from build123d import *

# Parameters (mm, degrees)
F0_R     = 3.175
F1_DEPTH = 3.048


with BuildPart() as f1:
    # F0 (on Front) → F1 (new body)
    with BuildSketch(Plane.XZ):
        with BuildLine():
            ThreePointArc((-9.4236638917, 68.6386150491), (-0.6947036893, 57.753275869), (9.525, 67.252908061))
            ThreePointArc((9.525, 67.252908061), (9.5066279666, 67.8442199118), (9.4515827392, 68.4332506914))
            ThreePointArc((9.4515827392, 68.4332506914), (0.1036267117, 76.7773443438), (-9.4236638917, 68.6386150491))
        make_face()
        with Locations((0, 67.252908061)):
            Circle(F0_R, mode=Mode.SUBTRACT)
        with BuildLine():
            ThreePointArc((9.4515827392, 68.4332506914), (9.5066279666, 67.8442199118), (9.525, 67.252908061))
            ThreePointArc((9.525, 67.252908061), (-0.6947036893, 57.753275869), (-9.4236638917, 68.6386150491))
            Line((-9.4236638917, 68.6386150491), (-17.0751139076, 16.6040263124))
            Line((-17.0751139076, 16.6040263124), (-9.4598263283, -48.1594366871))
            ThreePointArc((-9.4598263283, -48.1594366871), (-0.5571262079, -37.5383993165), (9.525, -47.047091939))
            ThreePointArc((9.525, -47.047091939), (6.9705567315, -53.5383910272), (0.6773435479, -56.5479777249))
            Line((0.6773435479, -56.5479777249), (44.7324052746, -54.9795665535))
            ThreePointArc((44.7324052746, -54.9795665535), (36.5125000006, -47.0471928378), (44.7322036046, -39.1146101473))
            Line((44.7322036046, -39.1146101473), (18.9234018404, -38.1964439189))
            ThreePointArc((18.9234018404, -38.1964439189), (13.2224661173, -35.485992741), (11.2938088242, -29.4753775685))
            Line((11.2938088242, -29.4753775685), (15.4327477068, 12.7318970133))
            ThreePointArc((15.4327477068, 12.7318970133), (-15.8733066778, 16.6847703328), (15.5348463028, 19.7215737442))
            Line((15.5348463028, 19.7215737442), (9.4515827392, 68.4332506914))
        make_face()
        with Locations((-3.175, 52.978108061)):
            Circle(F0_R, mode=Mode.SUBTRACT)
        with BuildLine():
            Line((15.8615962708, 17.1051263858), (15.5348463028, 19.7215737442))
            ThreePointArc((15.5348463028, 19.7215737442), (-15.8733066778, 16.6847703328), (15.4327477068, 12.7318970133))
            Line((15.4327477068, 12.7318970133), (15.8615962708, 17.1051263858))
        make_face()
        with Locations((0, 16.452908061)):
            Circle(F0_R, mode=Mode.SUBTRACT)
        with BuildLine():
            ThreePointArc((15.8615962708, 17.1051263858), (15.7526378986, 18.4201457783), (15.5348463028, 19.7215737442))
            Line((15.5348463028, 19.7215737442), (15.8615962708, 17.1051263858))
        make_face()
        with BuildLine():
            ThreePointArc((15.875, 16.452908061), (15.871648714, 16.7790860811), (15.8615962708, 17.1051263858))
            Line((15.8615962708, 17.1051263858), (15.4327477068, 12.7318970133))
            ThreePointArc((15.4327477068, 12.7318970133), (15.7640492077, 14.5793078964), (15.875, 16.452908061))
        make_face()
        with BuildLine():
            ThreePointArc((9.525, -47.047091939), (-0.5571262079, -37.5383993165), (-9.4598263283, -48.1594366871))
            ThreePointArc((-9.4598263283, -48.1594366871), (-6.329713314, -54.1647006921), (0, -56.572091939))
            Line((0, -56.572091939), (0.6773435479, -56.5479777249))
            ThreePointArc((0.6773435479, -56.5479777249), (6.9705567315, -53.5383910272), (9.525, -47.047091939))
        make_face()
        with Locations((0, -47.047091939)):
            Circle(F0_R, mode=Mode.SUBTRACT)
        with BuildLine():
            Line((0.6773435479, -56.5479777249), (0, -56.572091939))
            ThreePointArc((0, -56.572091939), (0.3388863295, -56.5660614764), (0.6773435479, -56.5479777249))
        make_face()
        with BuildLine():
            ThreePointArc((52.3875, -47.047091939), (50.1615627179, -41.5351088503), (44.7322036046, -39.1146101473))
            ThreePointArc((44.7322036046, -39.1146101473), (36.5125000006, -47.0471928378), (44.7324052746, -54.9795665535))
            ThreePointArc((44.7324052746, -54.9795665535), (50.1616327839, -52.5590024237), (52.3875, -47.047091939))
        make_face()
        with Locations((44.45, -47.047091939)):
            Circle(F0_R, mode=Mode.SUBTRACT)
    extrude(amount=F1_DEPTH)


solid = f1.part
Can you work these out from the model? Positions are in its coordinate system, mm. A direction names the side the tool comes from. Coordinates: 2 decimals unless noted, no trailing zeros. Write each loop counter-clockwise with the first axis right and the second up, starting at its lowest first coordinate (ties: lowest second). Pieces come first, ordered by that corner, then holes. Notation, with made-up numbers: (20, 58.25) -> (72, 58.25) arc R21 cw to (72, 79.25) -> close; hole circle Ø6 at (-19, 45.25). An arc over 180 degrees is marked (long way). Write item = value, one per line.
(1) On a 3-axis mill with a long thin cutter (end or side, diameter ignored), from which of +Z, -Z, +X, -X, +Y, -Y can I reach the whole of each face in a straight line? I mean faces 5 (the face through (13.334, -1.503, -8.667)), 6 (the face through (-13.196, -1.503, 42.986)). Say none if no direction works.
Verdict:
face_5 = +X, +Y, -Y
face_6 = +Z, -X, +Y, -Y
(2) Imagine slicing it at A-A (y = -1.4). State how many separate pieces and enclosed holes the cut face has, and give its area (3 significant figures).
Verdict:
separate_pieces = 1
enclosed_holes = 5
area = 3,830 mm^2
(3) If I drill on probe 1 along X at (y, z) = (-2.1, -49.5); probe 2 along X at (y, z) = (-1.25, -45.5); probe 3 along X at (y, z) = (-1, -31.5), over which ranges is the centre line in solid material (lowest first)?
Verdict:
probe_1 = -9.2 to -2.02, 2.02 to 42.43, 46.47 to 52
probe_2 = -9.77 to -2.77, 2.77 to 41.68, 47.22 to 52.24
probe_3 = -11.42 to 11.35
(4) Imagine slicing it at C-C (z = 9). Please give me the cut outline in (x, y), and give its area (3 significant figures).
Verdict:
outline = (-16.18, -3.05) -> (15.07, -3.05) -> (15.07, 0) -> (-16.18, 0) -> close
area = 95.2 mm^2
(5) For pin 1 (8.5 mm diameter, centred on x = 44.45, z = -47.05, fed in from +Y); pin 2 (5.5 mm diameter, centred on x = 0, z = -47.05, fed in from +Y), each with a flat end and sliding along its axis, tell me the tip position at first contact or that it passes through.
Verdict:
pin_1 = 0
pin_2 = through
(6) Thinking about a two-plate mould opening in X: for faces 1 (the face through (0.295, -1.503, 76.773)), 2 (the face through (12.536, -1.503, 43.736)), 3 (the face through (-0.688, -1.503, -50.147)), 4 (the face through (-13.32, -1.5, -15.32)), which applies, +X half, -X half, draft (parallel to the pull), parting line (faces both ways), or undercut?
Verdict:
face_1 = parting line
face_2 = +X half
face_3 = undercut
face_4 = -X half
(7) Imagine slicing it at B-B (x = -11). Please give me the cut outline in (y, z).
Verdict:
outline = (-3.05, -35.06) -> (0, -35.06) -> (0, 57.92) -> (-3.05, 57.92) -> close
